from build123d import *

# Parameters (mm, degrees)
STOCK_HORN_DRIVE_FLANGE_START       = 40
STOCK_HORN_DRIVE_FLANGE_PROFILE_R   = 12
STOCK_HORN_DRIVE_FLANGE_PROFILE_R_2 = 1.75
STOCK_HORN_DRIVE_FLANGE_DEPTH       = 3
D_COUPLING_RING_START               = 43
D_COUPLING_RING_PROFILE_R           = 7
D_COUPLING_RING_PROFILE_R_2         = 4.05
D_COUPLING_RING_DEPTH               = 5
D_KEY_LAND_START                    = 43
D_KEY_LAND_PROFILE_W                = 2.9
D_KEY_LAND_PROFILE_H                = 4.8
D_KEY_LAND_DEPTH                    = 5
STOCK_HORN_SCREWS_START             = 39
STOCK_HORN_SCREWS_PROFILE_R         = 1.1
STOCK_HORN_SCREWS_DEPTH             = 12.911688245


with BuildPart() as part:
    # Stock_horn_drive_flange_profile → Stock_horn_drive_flange (new body)
    with BuildSketch(Plane(origin=(0, 0, 0), x_dir=(1, 0, 0), z_dir=(0, 1, 0)).offset(STOCK_HORN_DRIVE_FLANGE_START)):
        with Locations(Location((0, 0, 0), (0, 0, 270))):
            Circle(STOCK_HORN_DRIVE_FLANGE_PROFILE_R)
        with Locations(Location((0, 0, 0), (0, 0, 270))):
            Circle(STOCK_HORN_DRIVE_FLANGE_PROFILE_R_2, mode=Mode.SUBTRACT)
    extrude(amount=STOCK_HORN_DRIVE_FLANGE_DEPTH)

    # D_coupling_ring_profile → D_coupling_ring (add)
    with BuildSketch(Plane(origin=(0, 0, 0), x_dir=(1, 0, 0), z_dir=(0, 1, 0)).offset(D_COUPLING_RING_START)):
        with Locations(Location((0, 0, 0), (0, 0, 270))):
            Circle(D_COUPLING_RING_PROFILE_R)
        with Locations(Location((0, 0, 0), (0, 0, 270))):
            Circle(D_COUPLING_RING_PROFILE_R_2, mode=Mode.SUBTRACT)
    extrude(amount=D_COUPLING_RING_DEPTH)

    # D_key_land_profile → D_key_land (add)
    with BuildSketch(Plane(origin=(0, 0, 0), x_dir=(1, 0, 0), z_dir=(0, 1, 0)).offset(D_KEY_LAND_START)):
        with Locations((4.55, 0)):
            Rectangle(D_KEY_LAND_PROFILE_W, D_KEY_LAND_PROFILE_H)
    extrude(amount=D_KEY_LAND_DEPTH)

    # Stock_horn_screws_profile → Stock_horn_screws (cut, through all)
    with BuildSketch(Plane(origin=(0, 0, 0), x_dir=(1, 0, 0), z_dir=(0, 1, 0)).offset(STOCK_HORN_SCREWS_START)):
        with Locations(Location((-8, 0, 0), (0, 0, 22.9239414))):
            Circle(STOCK_HORN_SCREWS_PROFILE_R)
        with Locations(Location((8, 0, 0), (0, 0, 157.0760586))):
            Circle(STOCK_HORN_SCREWS_PROFILE_R)
        with Locations(Location((0, -8, 0), (0, 0, 67.0760586))):
            Circle(STOCK_HORN_SCREWS_PROFILE_R)
        with Locations(Location((0, 8, 0), (0, 0, 292.9239414))):
            Circle(STOCK_HORN_SCREWS_PROFILE_R)
    extrude(amount=STOCK_HORN_SCREWS_DEPTH, mode=Mode.SUBTRACT)


solid = part.part
Verification items for the finished model (mm, model axes). A direction names the side the tool comes from. Round coordinates to 2 decimals unless told otherwise and drop trailing zeros. Order: outer loops, then holes, each group sorted by start corner. A loop starts at its lowest first (then second) coordinate and runs counter-clockwise, first axis right, second up. Notation, with made-up numbers: (31, 43.5) -> (36, 43.5) arc R16 cw to (36, 73.5) -> close; hole circle Ø1 at (80, 87). An arc over 180 degrees is marked (long way). Put each result on its own line as item: value.
1) Depth check by flat-ended pin: pin 1 (3 mm diameter, centred on x = -9, z = -9.5, fed in from +Y); pin 2 (1 mm diameter, centred on x = -7.5, y = 41, fed in from +Z); pin 3 (3 mm diameter, centred on x = -3.5, y = 44, fed in from -Z). Enter the tip coordinate at first touch or a pass-through.
Final values:
pin 1: stops at y = 43
pin 2: stops at z = 9.75
pin 3: stops at z = -11.76
2) Material ranges on line 1 (X direction, y = 41.8, z = 0); line 2 (Z direction, x = 0, y = 44); line 3 (Z direction, x = 0.5, y = 41), recorded low to high.
Final values:
line 1: x = -12 to -9.1, -6.9 to -1.75, 1.75 to 6.9, 9.1 to 12
line 2: z = -6.9 to -4.05, 4.05 to 6.9
line 3: z = -11.99 to -8.98, -7.02 to -1.68, 1.68 to 7.02, 8.98 to 11.99
3) Section check B-B (z = 0). Record the cut outline in (x, y), then the cut area to 4 significant figures.
Final values:
outline: (-12, 40) -> (-9.1, 40) -> (-9.1, 43) -> (-12, 43) -> close; (-6.9, 40) -> (-1.75, 40) -> (-1.75, 43) -> (-4.05, 43) -> (-4.05, 48) -> (-6.9, 48) -> close; (1.75, 40) -> (6.9, 40) -> (6.9, 48) -> (3.1, 48) -> (3.1, 43) -> (1.75, 43) -> close; (9.1, 40) -> (12, 40) -> (12, 43) -> (9.1, 43) -> close
area: 81.55 mm^2
4) Section check D-D (z = 8). Record the cut outline in (x, y).
Final values:
outline: (-8.94, 40) -> (-1.1, 40) -> (-1.1, 43) -> (-8.94, 43) -> close; (1.1, 40) -> (8.94, 40) -> (8.94, 43) -> (1.1, 43) -> close
5) Section check A-A (x = 0). Record the cut outline in (y, z).
Final values:
outline: (40, -12) -> (43, -12) -> (43, -9.1) -> (40, -9.1) -> close; (40, -6.9) -> (48, -6.9) -> (48, -4.05) -> (43, -4.05) -> (43, -1.75) -> (40, -1.75) -> close; (40, 1.75) -> (43, 1.75) -> (43, 4.05) -> (48, 4.05) -> (48, 6.9) -> (40, 6.9) -> close; (40, 9.1) -> (43, 9.1) -> (43, 12) -> (40, 12) -> close
6) Section check C-C (y = 47.25). Record the cut outline in (x, z), then the cut area to 3 significant figures.
Final values:
outline: (-6.99, -0.43) arc R7 ccw to (-0.43, -6.99) arc R1.1 cw to (0.43, -6.99) arc R7 ccw to (6.99, -0.43) arc R1.1 cw to (6.99, 0.43) arc R7 ccw to (0.43, 6.99) arc R1.1 cw to (-0.43, 6.99) arc R7 ccw to (-6.99, 0.43) arc R1.1 cw to start; hole (3.1, -2.4) -> (3.1, 2.4) -> (3.26, 2.4) arc R4.05 ccw (long way) to (3.26, -2.4) -> close
area: 106 mm^2
7) Set-up check for faces 4 (the flat face through (-5.2, 43, 5.2)), 5 (the cylindrical face through (-4.9, 45.5, -5)), 6 (the cylindrical face through (5, 45.5, -4.9)), 7 (the cylindrical face through (4.9, 45.5, 5)): record each of +Z, -Z, +X, -X, +Y, -Y from which the full face is reachable in a straight line by a thin tool's end or side.
Final values:
face 4: +Y
face 5: -Z, -X, +Y
face 6: -Z, +X, +Y
face 7: +Z, +X, +Y
8) Mould release check, pull along X, two halves, no side actions. Record for faces 1 (the cylindrical face through (0.104, 42.166, 6.905)), 2 (the cylindrical face through (3.604, 41.479, 11.446)), 3 (the cylindrical face through (-5, 45.5, 4.9)): +X half, -X half, draft (parallel to the pull), parting line (faces both ways), or undercut.
Final values:
face 1: undercut
face 2: parting line
face 3: -X half
